Build history of the part. All positions in model axes, mm. A direction names the side the tool comes from. Round coordinates to 2 decimals unless told otherwise and drop trailing zeros. Order: outer loops, then holes, each group sorted by start corner. A loop starts at its lowest first (then second) coordinate and runs counter-clockwise, first axis right, second up. Notation, with made-up numbers: (67, -33.75) - (113, -33.75) arc R7 ccw to (113, -28.75) - close; hole circle Ø11 at (36, 32.5). An arc over 180 degrees is marked (long way). Write each question's results on one line, items separated by ' | '. Start each with the question number.
```python
from build123d import *

# Parameters (mm, degrees)
SKETCH1_W                = 15.24
SKETCH1_H                = 30.9118
BOSS_EXTRUDE1_DEPTH      = 31.115
SKETCH2_W                = 15.24
SKETCH2_H                = 6.096
BOSS_EXTRUDE2_DEPTH      = 6.9215
BOSS_EXTRUDE2_DEPTH_BACK = 37.9095
SKETCH3_R                = 5.2705
BOSS_EXTRUDE3_DEPTH      = 3.9624
SKETCH4_R                = 6.3119
BOSS_EXTRUDE4_DEPTH      = 2.5019
SKETCH5_R                = 3.99415
BOSS_EXTRUDE5_DEPTH      = 2.3622
SKETCH6_R                = 8.4455
BOSS_EXTRUDE6_DEPTH      = 1.651
SKETCH7_R                = 3.5433
BOSS_EXTRUDE7_DEPTH      = 2.1844
CUT_EXTRUDE1_REACH       = 27.4
SKETCH8_R                = 1.5621
CUT_EXTRUDE2_REACH       = 27.4
SKETCH9_R                = 1.5621


with BuildPart() as part:
    # Sketch1 → Boss-Extrude1 (new body)
    with BuildSketch(Plane(origin=(0, 0, 0), x_dir=(1, 0, 0), z_dir=(0, 1, 0))):
        with Locations((7.62, 15.4559)):
            Rectangle(SKETCH1_W, SKETCH1_H)
    extrude(amount=BOSS_EXTRUDE1_DEPTH)

    # Sketch2 → Boss-Extrude2 (add, two sides)
    with BuildSketch(Plane.XY) as boss_extrude2_sk:
        with Locations((7.62, 22.352)):
            Rectangle(SKETCH2_W, SKETCH2_H)
    extrude(amount=BOSS_EXTRUDE2_DEPTH)
    extrude(boss_extrude2_sk.sketch, amount=-BOSS_EXTRUDE2_DEPTH_BACK)

    # Sketch3 → Boss-Extrude3 (add)
    with BuildSketch(Plane(origin=(0, 0, -30.9118), x_dir=(-1, 0, 0), z_dir=(0, 0, -1))):
        with Locations((-7.62, 8.2804)):
            Circle(SKETCH3_R)
    extrude(amount=BOSS_EXTRUDE3_DEPTH)

    # Sketch4 → Boss-Extrude4 (add)
    with BuildSketch(Plane(origin=(0, 31.115, 0), x_dir=(1, 0, 0), z_dir=(0, 1, 0))):
        with Locations((7.62, 24.2951)):
            Circle(SKETCH4_R)
    extrude(amount=BOSS_EXTRUDE4_DEPTH)

    # Sketch5 → Boss-Extrude5 (add)
    with BuildSketch(Plane(origin=(0, 33.6169, 0), x_dir=(1, 0, 0), z_dir=(0, 1, 0))):
        with Locations((7.62, 24.2951)):
            Circle(SKETCH5_R)
    extrude(amount=BOSS_EXTRUDE5_DEPTH)

    # Sketch6 → Boss-Extrude6 (add)
    with BuildSketch(Plane(origin=(0, 35.9791, 0), x_dir=(1, 0, 0), z_dir=(0, 1, 0))):
        with Locations((7.62, 24.2951)):
            Circle(SKETCH6_R)
    extrude(amount=BOSS_EXTRUDE6_DEPTH)

    # Sketch7 → Boss-Extrude7 (add)
    with BuildSketch(Plane(origin=(0, 37.6301, 0), x_dir=(1, 0, 0), z_dir=(0, 1, 0))):
        with Locations((7.62, 24.2951)):
            Circle(SKETCH7_R)
    extrude(amount=BOSS_EXTRUDE7_DEPTH)

    # Sketch8 → Cut-Extrude1 (cut, up to next)
    with BuildSketch(Plane(origin=(0, 25.4, 0), x_dir=(1, 0, 0), z_dir=(0, 1, 0)), mode=Mode.PRIVATE) as cut_extrude1_sk1:
        with Locations((7.62, -3.46075)):
            Circle(SKETCH8_R)
    cut_extrude1_tool1 = extrude(cut_extrude1_sk1.sketch, amount=-CUT_EXTRUDE1_REACH, mode=Mode.PRIVATE) & part.part
    add(cut_extrude1_tool1.solids().sort_by_distance((7.62, 25.4, 3.46075))[0], mode=Mode.SUBTRACT)

    # Sketch9 → Cut-Extrude2 (cut, up to next)
    with BuildSketch(Plane(origin=(0, 25.4, 0), x_dir=(1, 0, 0), z_dir=(0, 1, 0)), mode=Mode.PRIVATE) as cut_extrude2_sk1:
        with Locations((7.62, 34.41065)):
            Circle(SKETCH9_R)
    cut_extrude2_tool1 = extrude(cut_extrude2_sk1.sketch, amount=-CUT_EXTRUDE2_REACH, mode=Mode.PRIVATE) & part.part
    add(cut_extrude2_tool1.solids().sort_by_distance((7.62, 25.4, -34.41065))[0], mode=Mode.SUBTRACT)


solid = part.part
```
1. Mould opens along Z. For faces 1 (the face through (8.341, 22.395, -33.025)), 2 (the face through (8, 10, 0)), 3 (the face through (8.306, 13.506, -32.865)), 4 (the face through (2.968, 32.348, -28.561)) say: pulls with the +Z half, pulls with the -Z half, needs draft (parallel to the pull), parting line crosses it, or undercut.
2. Flat gauge pins, fed straight in: pin 1 Ø2 at (x, z) = (8, 4) entering from -Y; pin 2 Ø15.5 at (y, z) = (17.5, -8) entering from +X; pin 3 Ø4 at (x, z) = (12.5, -10) entering from +Y (3 decimals). Where does each tip first touch, or does it go through?
3. Cut at C-C (y = 24.5). List the corners of the cut face in (x, z).
4. Cut at D-D (y = 6). List the corners of the cut face in (x, z), plus the area to 3 significant figures.
5. Wall check: line 1 (Z direction, x = 7.62, y = 22.5); line 2 (Y direction, x = 11.5, z = -18) (3 decimals); line 3 (Y direction, x = 9.75, z = -18.5). Give the ranges that are in metal, low to high. Write a range as from..to.
6. Cut at A-A (x = 7.62). Give the number of separate pieces and of enclosed holes in the cut face, plus the area to 3 significant figures.
7. 3-axis set-ups, long thin cutter, end or side, ignore diameter. For faces 5 (the face through (8, 8, -34.874)), 6 (the face through (8, 33.617, -20)), 7 (the face through (5.8, 19.304, 3.4)): which of +Z, -Z, +X, -X, +Y, -Y reach the whole face in a straight line?
8. Cut at B-B (z = -29.5). List the corners of the cut face in (x, y) (3 decimals), plus the area to 3 significant figures.
A:
1) face 1: undercut | face 2: pulls with the +Z half | face 3: needs draft | face 4: parting line crosses it
2) pin 1: stops at y = 19.3 | pin 2: stops at x = 15.24 | pin 3: stops at y = 31.115
3) outline: (0, -37.91) - (15.24, -37.91) - (15.24, 6.92) - (0, 6.92) - close; hole circle Ø3.12 at (7.62, -34.41); hole circle Ø3.12 at (7.62, 3.46)
4) outline: (0, -30.91) - (2.87, -30.91) - (2.87, -34.87) - (12.37, -34.87) - (12.37, -30.91) - (15.24, -30.91) - (15.24, 0) - (0, 0) - close | area: 509 mm^2
5) line 1: z = -37.91..-35.97, -32.85..1.9, 5.02..6.92 | line 2: y = 0..31.115, 35.979..37.63 | line 3: y = 0..33.62, 35.98..37.63
6) separate pieces: 3 | enclosed holes: 0 | area: 1,140 mm^2
7) face 5: -Z, +X, -X, -Y | face 6: none | face 7: +Z, +X, -X, -Y
8) outline: (0, 0) - (15.24, 0) - (15.24, 31.115) - (11.191, 31.115) - (11.191, 33.617) - (4.049, 33.617) - (4.049, 31.115) - (0, 31.115) - close; (0.969, 35.979) - (14.271, 35.979) - (14.271, 37.63) - (0.969, 37.63) - close | area: 514 mm^2
